Design review of the part built by this model. Coordinates are the model's own, in mm. Face numbers are marked on the shaded views. A direction names the side the tool comes from. Round coordinates to 2 decimals unless told otherwise and drop trailing zeros. Order: outer loops, then holes, each group sorted by start corner. A loop starts at its lowest first (then second) coordinate and runs counter-clockwise, first axis right, second up. Notation, with made-up numbers: M -25,-21.5 L 1,-21.5 A21 ccw 1,16.5 Z; hole C 32.25,52 d2. An arc over 180 degrees is marked long. Use a Markdown table: item, result. Add a question column.
(1) Take a section at D-D (y = 8.5). Write out the cut boundary in (x, z).
(2) To check wall thickness, follow probe 1 along Z at (x, y) = (4.6, 12.75); probe 2 along X at (y, z) = (1.4, 24.7); probe 3 along Z at (x, y) = (3.45, 1.15). State the ranges of each line that lie inside material, in increasing order. Write a range as from..to.
(3) Take a section at C-C (x = 17.7). Write out the cut boundary in (y, z).
(4) For pin 1 (8 mm diameter, centred on y = 4, z = 21.5, fed in from -X); pin 2 (1 mm diameter, centred on x = 16, y = 10, fed in from -Z); pin 3 (4 mm diameter, centred on x = 4.6, z = 37.7, fed in from -Y); pin 4 (3 mm diameter, centred on x = 32.5, z = 24.5, fed in from +Y), all flat-tipped, find the tip position at first contact; note any pin that passes through.
(5) Machinability: for the marked faces 4, 5 and 6, which of the approach directions +Z, -Z, +X, -X, +Y, -Y give a long, thin tool a straight path to every point of the face, cutting with its end or side? Answer none if there is none.
(6) The part is to be moulded in two halves that separate along X. For the marked faces 1, 2 and 3, say which applies: released by +X, released by -X, zero draft, split by the parting line, or undercut.
(7) Take a section at A-A (y = 13.25). Write out the cut boundary in (x, z), then the cut area to 3 significant figures.
(8) Take a section at B-B (z = 37.7). Write out the cut boundary in (x, y).
```python
from build123d import *

# Parameters (mm, degrees)
F1_DEPTH  = 42.7
F3_DEPTH  = 4.5
F5_DEPTH  = 6
F6_R      = 8
F7_DEPTH  = 50
F8_R      = 11.7
F9_DEPTH  = 40
F10_R     = 1.75
F11_DEPTH = 25
F12_R     = 1.75
F13_DEPTH = 13
F14_R     = 1.75
F15_DEPTH = 13
F16_R     = 1.75
F17_DEPTH = 25
F18_R     = 1.75
F19_DEPTH = 7.5


with BuildPart() as f1:
    # F0 (on Top) → F1 (new body)
    with BuildSketch(Plane.XY):
        Polygon((0, 15.7), (0, 0), (35.4, 0), (35.4, 15.7), (23.2, 15.7), (7.2, 15.7), align=None)
    extrude(amount=F1_DEPTH)

    # F2 (on face) → F3 (cut)
    with BuildSketch(Plane.XY.offset(42.7)):
        with BuildLine():
            ThreePointArc((9.7, 15.7), (17.7, 7.7), (25.7, 15.7))
            Line((25.7, 15.7), (9.7, 15.7))
        make_face()
    extrude(amount=-F3_DEPTH, mode=Mode.SUBTRACT)

    # F4 (on face) → F5 (cut)
    with BuildSketch(Plane.XY.offset(38.2)):
        with BuildLine():
            ThreePointArc((11.45, 15.7), (17.7, 9.45), (23.95, 15.7))
            Line((23.95, 15.7), (11.45, 15.7))
        make_face()
    extrude(amount=-F5_DEPTH, mode=Mode.SUBTRACT)

    # F6 (on face) → F7 (cut)
    with BuildSketch(Plane.XY.offset(32.2)):
        with Locations((17.7, 15.7)):
            Circle(F6_R)
    extrude(amount=-F7_DEPTH, mode=Mode.SUBTRACT)

    # F8 (on face) → F9 (cut)
    with BuildSketch(Plane(origin=(0, 0, 32.2), x_dir=(1, 0, 0), z_dir=(0, 0, -1))):
        with Locations((17.7, -15.7)):
            Circle(F8_R)
    extrude(amount=F9_DEPTH, mode=Mode.SUBTRACT)

    # F10 (on face) → F11 (cut)
    with BuildSketch(Plane.XZ):
        with Locations((3.45, 24.7)):
            Circle(F10_R)
        with Locations((31.95, 24.7)):
            Circle(F10_R)
    extrude(amount=-F11_DEPTH, mode=Mode.SUBTRACT)

    # F12 (on face) → F13 (cut)
    with BuildSketch(Plane(origin=(0, 15.7, 0), x_dir=(-1, 0, 0), z_dir=(0, 1, 0))):
        with BuildLine():
            Line((-29.4, 23.1196519371), (-29.4, 26.2803480629))
            ThreePointArc((-29.4, 26.2803480629), (-34.95, 24.7), (-29.4, 23.1196519371))
        make_face()
        with Locations((-31.95, 24.7)):
            Circle(F12_R, mode=Mode.SUBTRACT)
        with BuildLine():
            ThreePointArc((-29.4, 23.1196519371), (-29.0646923907, 23.8784161637), (-28.95, 24.7))
            ThreePointArc((-28.95, 24.7), (-29.0646923907, 25.5215838363), (-29.4, 26.2803480629))
            Line((-29.4, 26.2803480629), (-29.4, 23.1196519371))
        make_face()
    extrude(amount=-F13_DEPTH, mode=Mode.SUBTRACT)

    # F14 (on face) → F15 (cut)
    with BuildSketch(Plane(origin=(0, 15.7, 0), x_dir=(-1, 0, 0), z_dir=(0, 1, 0))):
        with BuildLine():
            Line((-6, 23.1196519371), (-6, 26.2803480629))
            ThreePointArc((-6, 26.2803480629), (-6.45, 24.7), (-6, 23.1196519371))
        make_face()
        with BuildLine():
            ThreePointArc((-6, 23.1196519371), (-2.6284161637, 21.8146923907), (-0.45, 24.7))
            ThreePointArc((-0.45, 24.7), (-2.6284161637, 27.5853076093), (-6, 26.2803480629))
            Line((-6, 26.2803480629), (-6, 23.1196519371))
        make_face()
        with Locations((-3.45, 24.7)):
            Circle(F14_R, mode=Mode.SUBTRACT)
    extrude(amount=-F15_DEPTH, mode=Mode.SUBTRACT)

    # F16 (on face) → F17 (cut)
    with BuildSketch(Plane(origin=(0, 15.7, 0), x_dir=(-1, 0, 0), z_dir=(0, 1, 0))):
        with Locations((-30.8, 37.7)):
            Circle(F16_R)
        with Locations((-4.6, 37.7)):
            Circle(F16_R)
    extrude(amount=-F17_DEPTH, mode=Mode.SUBTRACT)

    # F18 (on face) → F19 (cut)
    with BuildSketch(Plane.XZ):
        Polygon((7.6, 35.9679491924), (7.6, 39.4320508076), (4.6, 41.1641016151), (1.6, 39.4320508076), (1.6, 35.9679491924), (4.6, 34.2358983849), align=None)
        with Locations((4.6, 37.7)):
            Circle(F18_R, mode=Mode.SUBTRACT)
        Polygon((27.8, 39.4320508076), (27.8, 35.9679491924), (30.8, 34.2358983849), (33.8, 35.9679491924), (33.8, 39.4320508076), (30.8, 41.1641016151), align=None)
        with Locations((30.8, 37.7)):
            Circle(F18_R, mode=Mode.SUBTRACT)
    extrude(amount=-F19_DEPTH, mode=Mode.SUBTRACT)


solid = f1.part
```
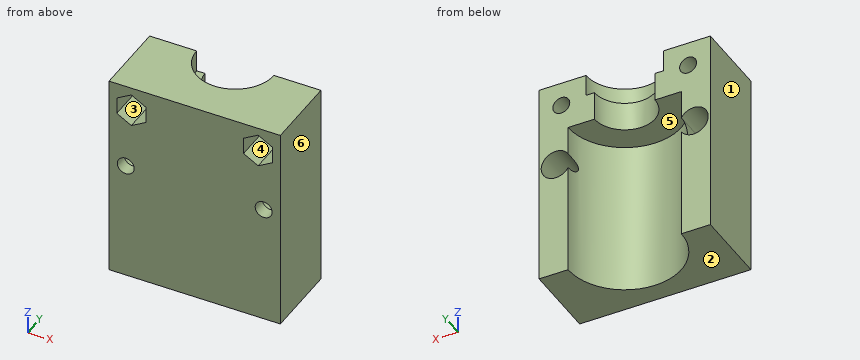
Verdict:
| question | item | result |
|---|---|---|
| 1 | outline | M 0,0 L 8.48,0 L 8.48,32.2 L 26.92,32.2 L 26.92,0 L 35.4,0 L 35.4,42.7 L 21.19,42.7 L 21.19,38.2 L 14.21,38.2 L 14.21,42.7 L 0,42.7 Z; hole C 3.45,24.7 d6; hole C 4.6,37.7 d3.5; hole C 31.95,24.7 d6; hole C 30.8,37.7 d3.5 |
| 2 | probe 1 | z = 0..21.93, 27.47..35.95, 39.45..42.7 |
| 2 | probe 2 | x = 0..1.7, 5.2..30.2, 33.7..35.4 |
| 2 | probe 3 | z = 0..22.95, 26.45..34.9, 40.5..42.7 |
| 3 | outline | M 0,0 L 4,0 L 4,32.2 L 9.45,32.2 L 9.45,38.2 L 7.7,38.2 L 7.7,42.7 L 0,42.7 Z |
| 4 | pin 1 | stops at x = 0 |
| 4 | pin 2 | stops at z = 32.2 |
| 4 | pin 3 | stops at y = 7.5 |
| 4 | pin 4 | stops at y = 2.7 |
| 5 | face 4 | -Y |
| 5 | face 5 | -Z, +Y |
| 5 | face 6 | +Z, -Z, +X, +Y, -Y |
| 6 | face 1 | released by -X |
| 6 | face 2 | zero draft |
| 6 | face 3 | undercut |
| 7 | outline | M 0,0 L 6.26,0 L 6.26,23.65 A3 cw long 6.26,25.75 L 6.26,32.2 L 11.95,32.2 L 11.95,38.2 L 10.08,38.2 L 10.08,42.7 L 0,42.7 Z; M 23.45,32.2 L 29.14,32.2 L 29.14,25.75 A3 cw long 29.14,23.65 L 29.14,0 L 35.4,0 L 35.4,42.7 L 25.32,42.7 L 25.32,38.2 L 23.45,38.2 Z; hole C 4.6,37.7 d3.5; hole C 30.8,37.7 d3.5 |
| 7 | area | 562 mm^2 |
| 8 | outline | M 0,0 L 1.6,0 L 1.6,7.5 L 2.85,7.5 L 2.85,15.7 L 0,15.7 Z; M 6.35,7.5 L 7.6,7.5 L 7.6,0 L 27.8,0 L 27.8,7.5 L 29.05,7.5 L 29.05,15.7 L 23.95,15.7 A6.25 cw 11.45,15.7 L 6.35,15.7 Z; M 32.55,7.5 L 33.8,7.5 L 33.8,0 L 35.4,0 L 35.4,15.7 L 32.55,15.7 Z |
